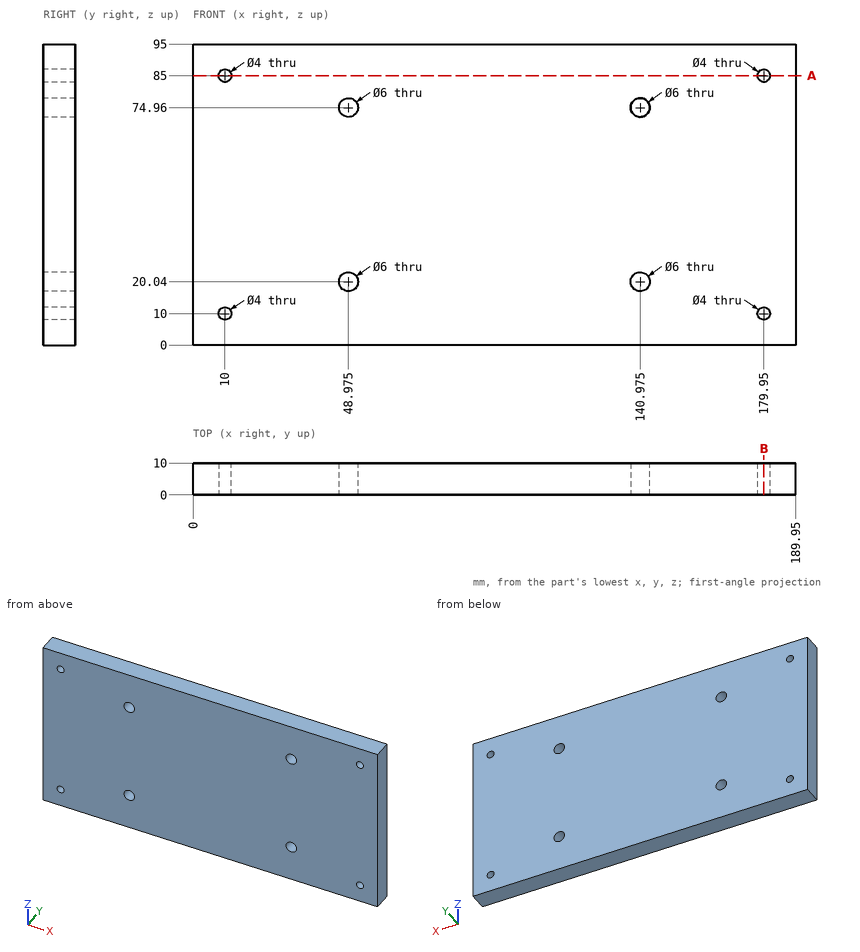
Job drawing, mm, ordinate dimensions from the low corner. One solid piece. Coordinates: 2 decimals unless noted, no trailing zeros. Order: outer loops, then holes, each group sorted by start corner. A loop starts at its lowest first (then second) coordinate and runs counter-clockwise, first axis right, second up. Notation, with made-up numbers: (5, -28) -> (61, -28) arc R21 cw to (61, -14) -> close; hole circle Ø5 at (84, 40.25). An arc over 180 degrees is marked (long way). Answer in a Markdown table with one row per item. Add a question column.
Q1. Band-saw the part on A-A, the plane z = 85. List the corners of the cut face in (x, y), then the cut area to 3 significant figures.
Q2. Wall check: line 1 along X through (y, z) = (4.5, 10); line 2 along Z through (x, y) = (179.95, 7.25); line 3 along X through (y, z) = (6.75, 85.5). Give the ranges that are in metal, low to high. Write a range as [from, to].
Q3. Band-saw the part on B-B, the plane x = 179.95. List the corners of the cut face in (y, z).
Answers follow:
| question | item | result |
|---|---|---|
| 1 | outline | (0, 0) -> (8, 0) -> (8, 10) -> (0, 10) -> close; (12, 0) -> (177.95, 0) -> (177.95, 10) -> (12, 10) -> close; (181.95, 0) -> (189.95, 0) -> (189.95, 10) -> (181.95, 10) -> close |
| 1 | area | 1,820 mm^2 |
| 2 | line 1 | [0, 8], [12, 177.95], [181.95, 189.95] |
| 2 | line 2 | [0, 8], [12, 83], [87, 95] |
| 2 | line 3 | [0, 8.06], [11.94, 178.01], [181.89, 189.95] |
| 3 | outline | (0, 0) -> (10, 0) -> (10, 8) -> (0, 8) -> close; (0, 12) -> (10, 12) -> (10, 83) -> (0, 83) -> close; (0, 87) -> (10, 87) -> (10, 95) -> (0, 95) -> close |
